Build history of the part. All positions in model axes, mm. A direction names the side the tool comes from. Round coordinates to 2 decimals unless told otherwise and drop trailing zeros. Write each loop counter-clockwise with the first axis right and the second up, starting at its lowest first coordinate (ties: lowest second). Pieces come first, ordered by that corner, then holes. Notation, with made-up numbers: M -34,89.5 L -16,89.5 A11 ccw -16,103.5 Z; hole C -3,-31 d2. An arc over 180 degrees is marked long. Write item = value, one per line.
from build123d import *

# Parameters (mm, degrees)
SKETCH_1_W                = 44.5
SKETCH_1_H                = 51
EXTRUDE_1_DEPTH           = 8
SKETCH_2_W                = 38
SKETCH_2_H                = 25
CUT_EXTRUDE_1_DEPTH       = 9
MM_1_D                    = 2.5
FILLET_1_R                = 1.5
SKETCH_5_W                = 37.2
SKETCH_5_H                = 20
CUT_EXTRUDE_2_DEPTH       = 15
SKETCH_6_W                = 6
SKETCH_6_H                = 8
EXTRUDE_2_DEPTH           = 5
HOLE_WIZARD_2_D           = 2.4
HOLE_WIZARD_2_CBORE_D     = 4.3
HOLE_WIZARD_2_CBORE_DEPTH = 2.3


with BuildPart() as part:
    # 草图1 → 凸台-拉伸1 (new body)
    with BuildSketch(Plane.XY):
        Rectangle(SKETCH_1_W, SKETCH_1_H)
    extrude(amount=EXTRUDE_1_DEPTH)

    # 草图2 → 切除-拉伸1 (cut, through all)
    with BuildSketch(Plane.XY.offset(8)):
        with Locations((0, 13)):
            Rectangle(SKETCH_2_W, SKETCH_2_H)
    extrude(amount=-CUT_EXTRUDE_1_DEPTH, mode=Mode.SUBTRACT)

    # 大小mm 暗销孔1 (through all)
    with Locations(Plane.ZY.offset(22.25)):
        with Locations((4, 21.5)):
            Hole(MM_1_D / 2)

    # 圆角1
    fillet_1_edges = [part.edges().sort_by_distance(p)[0] for p in [
        (20.625, 25.5, 8),
        (-20.625, 25.5, 0),
        (-20.625, 25.5, 8),
        (20.625, 25.5, 0),
    ]]
    fillet(fillet_1_edges, radius=FILLET_1_R)

    # 草图5 → 切除-拉伸2 (cut)
    with BuildSketch(Plane(origin=(0, 0, 0), x_dir=(-1, 0, 0), z_dir=(0, 0, -1))):
        with Locations((0, -15.5)):
            Rectangle(SKETCH_5_W, SKETCH_5_H)
    extrude(amount=-CUT_EXTRUDE_2_DEPTH, mode=Mode.SUBTRACT)

    # 草图6 → 凸台-拉伸2 (add)
    with BuildSketch(Plane.XZ.offset(25.5)):
        with Locations((-25.25, 4)):
            Rectangle(SKETCH_6_W, SKETCH_6_H)
    extrude_2 = extrude(amount=-EXTRUDE_2_DEPTH)

    # 镜向1: 凸台-拉伸2 across plane
    add(extrude_2.mirror(Plane(origin=(0, 0, 0), x_dir=(0, 0, 1), z_dir=(1, 0, 0))))

    # 打孔尺寸(%根据)内六角圆柱头螺钉的类型2 (through all)
    with Locations(Plane(origin=(0, -20.5, 0), x_dir=(1, 0, 0), z_dir=(0, 1, 0))):
        with Locations((-25.25, -4)):
            hole_wizard_2 = CounterBoreHole(HOLE_WIZARD_2_D / 2, HOLE_WIZARD_2_CBORE_D / 2, HOLE_WIZARD_2_CBORE_DEPTH)

    # 镜向2: 打孔尺寸(%根据)内六角圆柱头螺钉的类型2 across plane
    add(hole_wizard_2.mirror(Plane(origin=(0, 0, 0), x_dir=(0, 0, 1), z_dir=(1, 0, 0))), mode=Mode.SUBTRACT)


solid = part.part
1. Probe probe 1 along X at (y, z) = (-24.3, 4); probe 2 along X at (y, z) = (-18, 2.5); probe 3 along X at (y, z) = (17.5, 1). List the from-to ranges inside material, lowest first.
Responses:
probe_1 = -28.25 to -26.45, -24.05 to -18.6, 18.6 to 24.05, 26.45 to 28.25
probe_2 = -22.25 to -18.6, 18.6 to 22.25
probe_3 = -22.25 to -19, 19 to 22.25
2. Tool access for faces 1 (the face through (-20.6, 20.28, 4.27)), 2 (the face through (-23.2, -21.63, 3.35)), 3 (the face through (19, 13, 4)), 4 (the face through (0, -5.5, 4)), 5 (the face through (-22.25, 2, 4)): list every direction of +Z, -Z, +X, -X, +Y, -Y with a clear straight run to the whole face (end or side of a thin tool).
Responses:
face_1 = +X, -X
face_2 = +Y
face_3 = +Z, -Z, +Y
face_4 = +Z, -Z, -Y
face_5 = +Z, -Z, -X, +Y
3. Mould opens along Z. For faces 6 (the face through (-2, -5, 8)), 7 (the face through (22.25, 2, 4)), 8 (the face through (-24, -22.8, 5)), 9 (the face through (-20.6, 25.05, 0.43)) say: pulls with the +Z half, pulls with the -Z half, needs draft (parallel to the pull), parting line crosses it, or undercut.
Responses:
face_6 = pulls with the +Z half
face_7 = needs draft
face_8 = undercut
face_9 = pulls with the -Z half
4. Band-saw the part on A-A (x = 25.25). List the corners of the cut face in (y, z).
Responses:
outline = M -25.5,0 L -20.5,0 L -20.5,1.85 L -22.8,1.85 L -22.8,2.8 L -25.5,2.8 Z; M -25.5,5.2 L -22.8,5.2 L -22.8,6.15 L -20.5,6.15 L -20.5,8 L -25.5,8 Z
5. Band-saw the part on C-C (y = 21.5). List the corners of the cut face in (x, z).
Responses:
outline = M -22.25,0 L -19,0 L -19,2.75 L -22.25,2.75 Z; M -22.25,5.25 L -19,5.25 L -19,8 L -22.25,8 Z; M 19,0 L 22.25,0 L 22.25,2.75 L 19,2.75 Z; M 19,5.25 L 22.25,5.25 L 22.25,8 L 19,8 Z
6. Flat gauge pins, fed straight in: pin 1 (1.8 mm diameter, centred on x = -26.5, z = 3.5, fed in from +Y); pin 2 (4 mm diameter, centred on x = 7.5, z = 3, fed in from +Y); pin 3 (2.5 mm diameter, centred on x = -9, z = 6, fed in from -Y). Where does each tip first touch, or does it go through?
Responses:
pin_1 = -20.5
pin_2 = 0.5
pin_3 = -5.5
7. Band-saw the part on B-B (y = -19). List the corners of the cut face in (x, z).
Responses:
outline = M -22.25,0 L -18.6,0 L -18.6,8 L -22.25,8 Z; M 18.6,0 L 22.25,0 L 22.25,8 L 18.6,8 Z
8. Band-saw the part on D-D (z = 4). Count the separate pieces of the cut face and the enclosed holes in it, plus the area to 3 significant figures.
Responses:
separate_pieces = 5
enclosed_holes = 0
area = 587 mm²
